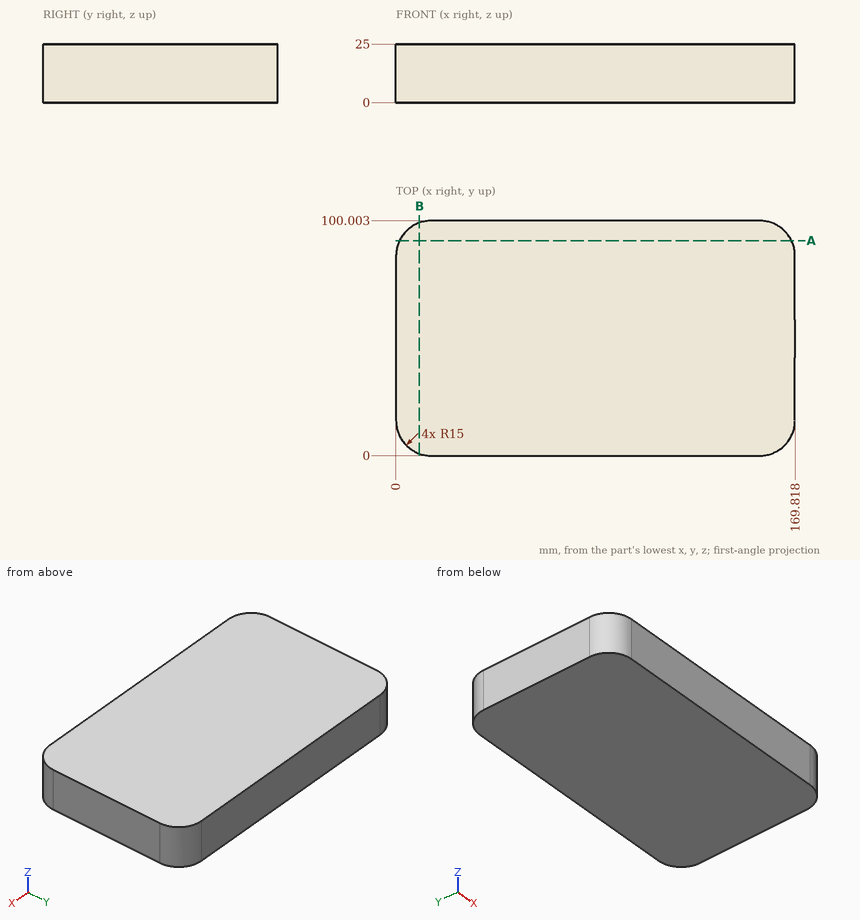
Check sheet for the drawn part. Datum: minimum x, y, z corner. Units: mm. Coordinates: 2 decimals unless noted, no trailing zeros. Order: outer loops, then holes, each group sorted by start corner. A loop starts at its lowest first (then second) coordinate and runs counter-clockwise, first axis right, second up. Notation, with made-up numbers: (60, 84.5) - (94, 84.5) arc R17 ccw to (94, 115.5) - close; hole circle Ø5 at (-28.5, 69.5). An arc over 180 degrees is marked (long way). Return JSON: item names as keys, results as strings.
(1) Thickness scan on line 1 along X through (y, z) = (91.5, 17.25); line 2 along Y through (x, z) = (7, 9); line 3 along X through (y, z) = (12, 3) (1 decimal). Record the ranges inside material, lowest first.
Filled sheet:
{"line 1": "x = 1.48 to 168.34", "line 2": "y = 2.31 to 97.69", "line 3": "x = 0.3 to 169.5"}
(2) Section check B-B, the plane x = 10. Record the cut outline in (y, z) (1 decimal), and give its area (3 significant figures).
Filled sheet:
{"outline": "(0.9, 0) - (99.1, 0) - (99.1, 25) - (0.9, 25) - close", "area": "2,460 mm^2"}
(3) Go/stop test with a flat-tipped pin: pin 1 (1.5 mm diameter, centred on y = 50, z = 6.5, fed in from -X). Record where the tip stops, or that it passes through.
Filled sheet:
{"pin 1": "stops at x = 0"}
(4) Section check A-A, the plane y = 91.5. Record the cut outline in (x, z), and give its area (3 significant figures).
Filled sheet:
{"outline": "(1.48, 0) - (168.34, 0) - (168.34, 25) - (1.48, 25) - close", "area": "4,170 mm^2"}
